```python
from build123d import *

# Parameters (mm, degrees)
BOSS_EXTRUDE1_DEPTH     = 25.4
CUT_EXTRUDE1_DEPTH      = 73.955945611
CUT_EXTRUDE1_DEPTH_BACK = 73.955945611
SKETCH2_R               = 2
SKETCH3_R               = 2.75
CUT_EXTRUDE2_DEPTH      = 73.955945755
CHAMFER1_SIZE           = 0.762


with BuildPart() as part:
    # Sketch1 → Boss-Extrude1 (new body)
    with BuildSketch(Plane.XY):
        with BuildLine():
            Line((0, 0), (67.202083301, 0))
            ThreePointArc((67.202083301, 0), (33.601041651, -12.7), (0, 0))
        make_face()
    extrude(amount=BOSS_EXTRUDE1_DEPTH)

    # Sketch2 → Cut-Extrude1 (cut, two sides: drawn at the far end of the back side and taken through both)
    with BuildSketch(Plane(origin=(0, 0, 0), x_dir=(1, 0, 0), z_dir=(0, 1, 0)).offset(-CUT_EXTRUDE1_DEPTH_BACK)):
        with Locations(Location((14.551041651, -12.7, 0), (0, 0, 270))):
            Circle(SKETCH2_R)
        with Locations(Location((52.651041651, -12.7, 0), (0, 0, 270))):
            Circle(SKETCH2_R)
    extrude(amount=CUT_EXTRUDE1_DEPTH + CUT_EXTRUDE1_DEPTH_BACK, mode=Mode.SUBTRACT)

    # Sketch3 → Cut-Extrude2 (cut, through all)
    with BuildSketch(Plane(origin=(0, 0, 0), x_dir=(1, 0, 0), z_dir=(0, 1, 0))):
        with Locations(Location((14.551041651, -12.7, 0), (0, 0, 270))):
            Circle(SKETCH3_R)
        with Locations(Location((52.651041651, -12.7, 0), (0, 0, 270))):
            Circle(SKETCH3_R)
    extrude(amount=-CUT_EXTRUDE2_DEPTH, mode=Mode.SUBTRACT)

    # Chamfer1
    chamfer1_edges = [part.edges().sort_by_distance(p)[0] for p in [
        (14.551041651, 0, 9.95),
        (52.651041651, 0, 9.95),
    ]]
    chamfer(chamfer1_edges, length=CHAMFER1_SIZE)


solid = part.part
```
CAD build for the part. Positions are in the model's coordinates, mm. Round coordinates to 2 decimals unless told otherwise and drop trailing zeros. Order: outer loops, then holes, each group sorted by start corner. A loop starts at its lowest first (then second) coordinate and runs counter-clockwise, first axis right, second up. Notation, with made-up numbers: (59, -23.75) -> (74, -23.75) arc R29 ccw to (74, 14.25) -> close; hole circle Ø10 at (-6.75, 39.5). An arc over 180 degrees is marked (long way). Write item = value, one per line.
(1) Cut at D-D (x = 8). Write the cut outline in (y, z), plus the area to 3 significant figures.
Answers follow:
outline = (-5.78, 0) -> (0, 0) -> (0, 25.4) -> (-5.78, 25.4) -> close
area = 147 mm²
(2) Cut at B-B (y = -5.75). Write the cut outline in (x, z), plus the area to 3 significant figures.
Answers follow:
outline = (7.95, 0) -> (59.25, 0) -> (59.25, 25.4) -> (7.95, 25.4) -> close; hole circle Ø5.5 at (14.55, 12.7); hole circle Ø5.5 at (52.65, 12.7)
area = 1,260 mm²
(3) Cut at A-A (z = 12.7). Write the cut outline in (x, y).
Answers follow:
outline = (0, 0) arc R50.8 ccw to (11.8, -7.78) -> (11.8, -0.76) -> (11.04, 0) -> close; (17.3, -10.01) arc R50.8 ccw to (49.9, -10.01) -> (49.9, -0.76) -> (49.14, 0) -> (18.06, 0) -> (17.3, -0.76) -> close; (55.4, -7.78) arc R50.8 ccw to (67.2, 0) -> (56.16, 0) -> (55.4, -0.76) -> close
(4) Flat gauge pins, fed straight in: P1, Ø6, axis at y = -7, z = 17.5, coming from the -X side; P2, Ø1.5, axis at y = -3.5, z = 21, coming from the -X side; P3, Ø5, axis at y = -10.5, z = 15, coming from the -X side; P4, Ø5, axis at x = 10.5, z = 18.5, coming from the +Y side. Where does each tip first touch, or does it go through?
Answers follow:
P1 = 5.17
P2 = 3.4
P3 = 12.26
P4 = 0
(5) Drill centre lines: L1, parallel to X at y = -1.25, z = 14; L2, parallel to X at y = -4, z = 12.7; L3, parallel to Z at x = 14, y = -4.25. Where is each one in solid material? Low to high.
Answers follow:
L1 = 1.47 to 12.13, 16.97 to 50.23, 55.07 to 65.73
L2 = 5.17 to 11.8, 17.3 to 49.9, 55.4 to 62.03
L3 = 0 to 10.01, 15.39 to 25.4
(6) Cut at C-C (z = 21). Write the cut outline in (x, y).
Answers follow:
outline = (0, 0) arc R50.8 ccw to (67.2, 0) -> close
(7) Pull direction Z, two halves, no side cores. Call faces 1 (the flat face through (33, 0, 13)), 2 (the flat face through (34, -5, 25.4)), 3 (the cylindrical face through (49.966, -5.331, 12.104)), 4 (the flat face through (34, -5, 0)): +Z half, -Z half, draft (parallel to the pull), parting line (faces both ways), or undercut.
Answers follow:
face_1 = draft
face_2 = +Z half
face_3 = undercut
face_4 = -Z half
